Part model, mm, in its own coordinate system. A direction names the side the tool comes from. Give positions to 0.01 mm unless a question says otherwise; leave off trailing zeros. Write each loop counter-clockwise with the first axis right and the second up, starting at its lowest first coordinate (ties: lowest second). Pieces come first, ordered by that corner, then holes. Notation, with made-up numbers: M 9.25,31 L 15.25,31 A15 cw 15.25,44 Z; hole C 32.25,45.25 d2. An arc over 180 degrees is marked long. Use a Markdown table: item, result. Add a question column.
from build123d import *

# Parameters (mm, degrees)
SKETCH1_W                = 14.05
SKETCH1_H                = 11.6
BOSS_EXTRUDE1_DEPTH      = 6.03
SKETCH2_W                = 5.95
SKETCH2_H                = 8.82
CUT_EXTRUDE2_DEPTH       = 6.03
SKETCH3_W                = 0.5
SKETCH3_H                = 4
BOSS_EXTRUDE2_DEPTH      = 6.03
M3_CLEARANCE_HOLE1_D     = 3.2
M3_CLEARANCE_HOLE1_DEPTH = 2.78


with BuildPart() as part:
    # Sketch1 → Boss-Extrude1 (new body)
    with BuildSketch(Plane.XY):
        Rectangle(SKETCH1_W, SKETCH1_H)
    extrude(amount=BOSS_EXTRUDE1_DEPTH)

    # Sketch2 → Cut-Extrude2 (cut)
    with BuildSketch(Plane.XY.offset(6.03)):
        with Locations((0, 1.39)):
            Rectangle(SKETCH2_W, SKETCH2_H)
    extrude(amount=-CUT_EXTRUDE2_DEPTH, mode=Mode.SUBTRACT)

    # Sketch3 → Boss-Extrude2 (add)
    with BuildSketch(Plane(origin=(-2.975, 0, 0), x_dir=(0, 0, -1), z_dir=(1, 0, 0))):
        with Locations((-3.015, 3.8)):
            Rectangle(SKETCH3_W, SKETCH3_H)
    extrude(amount=BOSS_EXTRUDE2_DEPTH)

    # M3 Clearance Hole1
    with Locations(Plane(origin=(0, -5.8, 0), x_dir=(-1, 0, 0), z_dir=(0, -1, 0))):
        with Locations((0, -3.015)):
            Hole(M3_CLEARANCE_HOLE1_D / 2, depth=M3_CLEARANCE_HOLE1_DEPTH)


solid = part.part
1. Cut at B-B (y = -0.25). Write the cut outline in (x, z) (3 decimals).
2. Flat gauge pins, fed straight in: pin 1 (1 mm diameter, centred on x = -0.5, y = -2, fed in from +Z); pin 2 (2 mm diameter, centred on x = 0.5, y = 3.5, fed in from +Z) (3 decimals). Where does each tip first touch, or does it go through?
3. Cut at A-A (x = 2). Write the cut outline in (y, z) (3 decimals).
4. Mould opens along X. For faces 1 (the flat face through (-3.2, 0.1, 0)), 2 (the cylindrical face through (-0.21, -4.39, 1.43)), 3 (the flat face through (-7.025, 0, 3)) say: released by +X, released by -X, zero draft, split by the parting line, or undercut.
5. Tool access for faces 4 (the flat face through (0, 4, 3.265)), 5 (the flat face through (-2, -5.8, 3)), 6 (the flat face through (0, 4, 2.765)): list every direction of +Z, -Z, +X, -X, +Y, -Y with a clear straight run to the whole face (end or side of a thin tool).
6. Cut at D-D (x = 0). Write the cut outline in (y, z) (3 decimals), then the cut area to 3 significant figures.
7. Drill centre lines: probe 1 along X at (y, z) = (-0.25, 4.5) (3 decimals); probe 2 along Z at (x, y) = (0, -4.8) (3 decimals); probe 3 along Y at (x, z) = (-0.5, 5.5). Where is each one in solid material? Low to high. Write a range as [from, to].
8. Cut at C-C (z = 0.5). Write the cut outline in (x, y) (3 decimals), then the cut area to 3 significant figures.
A:
| question | item | result |
|---|---|---|
| 1 | outline | M -7.025,0 L -2.975,0 L -2.975,6.03 L -7.025,6.03 Z; M 2.975,0 L 7.025,0 L 7.025,6.03 L 2.975,6.03 Z |
| 2 | pin 1 | passes through |
| 2 | pin 2 | stops at z = 3.265 |
| 3 | outline | M -5.8,0 L -3.02,0 L -3.02,6.03 L -5.8,6.03 Z; M 1.8,2.765 L 5.8,2.765 L 5.8,3.265 L 1.8,3.265 Z |
| 4 | face 1 | zero draft |
| 4 | face 2 | undercut |
| 4 | face 3 | released by -X |
| 5 | face 4 | +Z, +Y |
| 5 | face 5 | +Z, -Z, +X, -X, -Y |
| 5 | face 6 | -Z, +Y |
| 6 | outline | M -5.8,0 L -3.02,0 L -3.02,1.415 L -5.8,1.415 Z; M -5.8,4.615 L -3.02,4.615 L -3.02,6.03 L -5.8,6.03 Z; M 1.8,2.765 L 5.8,2.765 L 5.8,3.265 L 1.8,3.265 Z |
| 6 | area | 9.87 mm² |
| 7 | probe 1 | x = [-7.025, -2.975], [2.975, 7.025] |
| 7 | probe 2 | z = [0, 1.415], [4.615, 6.03] |
| 7 | probe 3 | y = [-5.8, -3.02] |
| 8 | outline | M -7.025,-5.8 L 7.025,-5.8 L 7.025,5.8 L 2.975,5.8 L 2.975,-3.02 L -2.975,-3.02 L -2.975,5.8 L -7.025,5.8 Z |
| 8 | area | 111 mm² |
